Here's how the part is built. I have some questions about the finished solid (model axes, mm). Face numbers are marked on the shaded views. A direction names the side the tool comes from. Give positions to 0.01 mm unless a question says otherwise; leave off trailing zeros. Order: outer loops, then holes, each group sorted by start corner. A loop starts at its lowest first (then second) coordinate and runs counter-clockwise, first axis right, second up.
from build123d import *

# Parameters (mm, degrees)
SKETCH_1_W               = 62
SKETCH_1_H               = 25
EXTRUDE_1_DEPTH          = 2
SKETCH_2_R               = 3
EXTRUDE_2_DEPTH          = 5
SKETCH_3_R               = 1.5
CUT_EXTRUDE_1_DEPTH      = 1
CUT_EXTRUDE_1_DEPTH_BACK = 8
SKETCH_4_R               = 2
CUT_EXTRUDE_2_DEPTH      = 6
CUT_EXTRUDE_2_DEPTH_BACK = 3
FILLET_1_R               = 2
FILLET_2_R               = 2
FILLET_3_R               = 2
FILLET_4_R               = 2


with BuildPart() as part:
    # Эскиз1 → Бобышка-Вытянуть1 (new body)
    with BuildSketch(Plane(origin=(0, 0, 0), x_dir=(1, 0, 0), z_dir=(0, 1, 0))):
        with Locations((31, -12.5)):
            Rectangle(SKETCH_1_W, SKETCH_1_H)
    extrude(amount=EXTRUDE_1_DEPTH)

    # Эскиз2 → Бобышка-Вытянуть2 (add)
    with BuildSketch(Plane(origin=(0, 2, 0), x_dir=(1, 0, 0), z_dir=(0, 1, 0))):
        with Locations((14.75, -4)):
            Circle(SKETCH_2_R)
        with Locations((47.5, -21)):
            Circle(SKETCH_2_R)
    extrude(amount=EXTRUDE_2_DEPTH)

    # Эскиз3 → Вырез-Вытянуть1 (cut, two sides)
    with BuildSketch(Plane(origin=(0, 7, 0), x_dir=(1, 0, 0), z_dir=(0, 1, 0))) as cut_extrude_1_sk:
        with Locations((14.75, -4)):
            Circle(SKETCH_3_R)
        with Locations((47.5, -21)):
            Circle(SKETCH_3_R)
    extrude(amount=CUT_EXTRUDE_1_DEPTH, mode=Mode.SUBTRACT)
    extrude(cut_extrude_1_sk.sketch, amount=-CUT_EXTRUDE_1_DEPTH_BACK, mode=Mode.SUBTRACT)

    # Эскиз4 → Вырез-Вытянуть2 (cut, two sides)
    with BuildSketch(Plane(origin=(0, 2, 0), x_dir=(1, 0, 0), z_dir=(0, 1, 0))) as cut_extrude_2_sk:
        with Locations((3, -12.5)):
            Circle(SKETCH_4_R)
        with Locations((59, -12.5)):
            Circle(SKETCH_4_R)
    extrude(amount=CUT_EXTRUDE_2_DEPTH, mode=Mode.SUBTRACT)
    extrude(cut_extrude_2_sk.sketch, amount=-CUT_EXTRUDE_2_DEPTH_BACK, mode=Mode.SUBTRACT)

    # Скругление1
    fillet_1_edges = [part.edges().sort_by_distance(p)[0] for p in [
        (0, 1, 0),
    ]]
    fillet(fillet_1_edges, radius=FILLET_1_R)

    # Скругление2
    fillet_2_edges = [part.edges().sort_by_distance(p)[0] for p in [
        (0, 1, 25),
    ]]
    fillet(fillet_2_edges, radius=FILLET_2_R)

    # Скругление3
    fillet_3_edges = [part.edges().sort_by_distance(p)[0] for p in [
        (62, 1, 25),
    ]]
    fillet(fillet_3_edges, radius=FILLET_3_R)

    # Скругление4
    fillet_4_edges = [part.edges().sort_by_distance(p)[0] for p in [
        (62, 1, 0),
    ]]
    fillet(fillet_4_edges, radius=FILLET_4_R)


solid = part.part
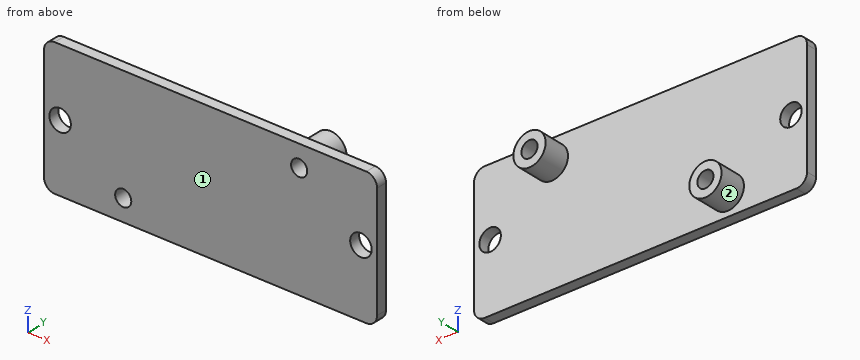
Q1. If we section it at C-C on z = 4: List the corners of the cut face in (x, y) for me.
Filled sheet:
outline: (0, 0) - (13.25, 0) - (13.25, 7) - (11.75, 7) - (11.75, 2) - (0, 2) - close; (16.25, 0) - (62, 0) - (62, 2) - (17.75, 2) - (17.75, 7) - (16.25, 7) - close
Q2. For the marked faces 1 and 2, which set-ups out of +Z, -Z, +X, -X, +Y, -Y let a thin tool reach every point of the face, with its end or its side?
Filled sheet:
face 1: +Z, -Z, +X, -X, -Y
face 2: +Y
Q3. I need wall thicknesses on L1, parallel to X at y = 0.65, z = 12.5; L2, parallel to X at y = 5.25, z = 21; L3, parallel to Z at x = 14.75, y = 3. Which ranges of each line are inside material? Lowest first, please.
Filled sheet:
L1: x = 0 to 1, 5 to 57, 61 to 62
L2: x = 44.5 to 46, 49 to 50.5
L3: z = 1 to 2.5, 5.5 to 7
Q4. If we section it at B-B on x = 59: List the corners of the cut face in (y, z) for me, plus the area to 3 significant figures.
Filled sheet:
outline: (0, 0) - (2, 0) - (2, 10.5) - (0, 10.5) - close; (0, 14.5) - (2, 14.5) - (2, 25) - (0, 25) - close
area: 42.0 mm2
Q5. If we section it at D-D on y = 5.5: List the corners of the cut face in (x, z) for me.
Filled sheet:
outline: circle Ø6 at (14.75, 4); circle Ø6 at (47.5, 21); hole circle Ø3 at (14.75, 4); hole circle Ø3 at (47.5, 21)
Q6. I'm going to push flat-ended pins straight in: P1, Ø4, axis at x = 47.5, z = 21, coming from the +Y side; P2, Ø1.5, axis at x = 26, y = 4, coming from the +Z side; P3, Ø4, axis at x = 15.5, z = 12, coming from the +Y side. Where does each tip first touch, or does it pass through?
Filled sheet:
P1: stops at y = 7
P2: passes through
P3: stops at y = 2
Q7. If we section it at A-A on z = 12.5: List the corners of the cut face in (x, y) for me.
Filled sheet:
outline: (0, 0) - (1, 0) - (1, 2) - (0, 2) - close; (5, 0) - (57, 0) - (57, 2) - (5, 2) - close; (61, 0) - (62, 0) - (62, 2) - (61, 2) - close
